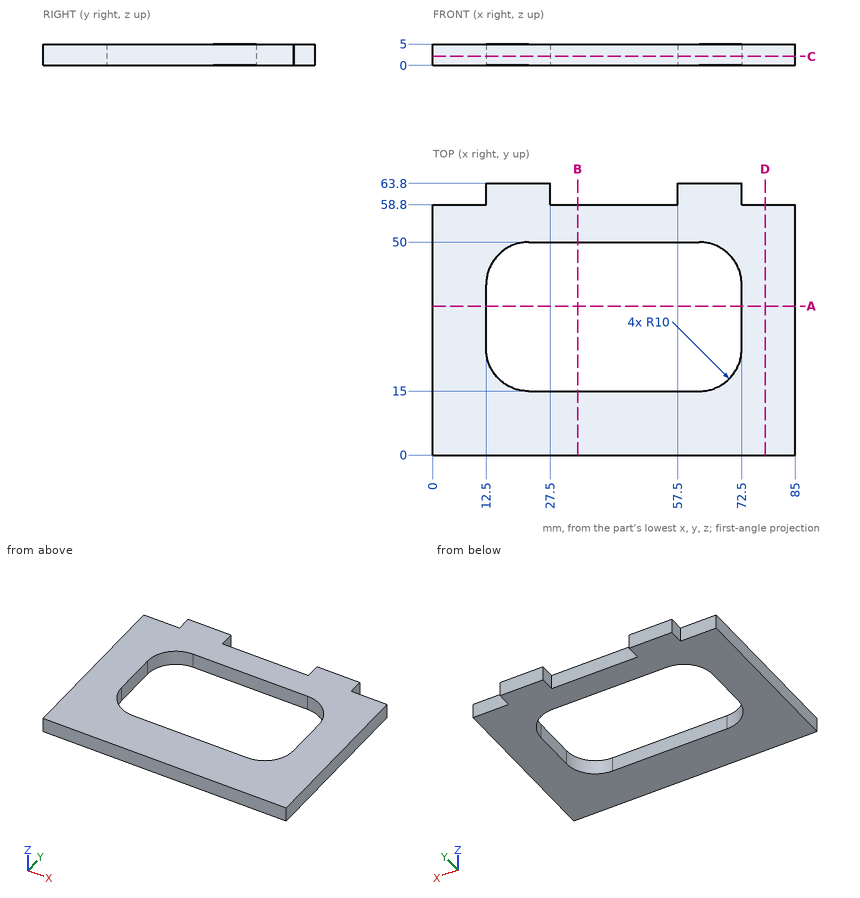
Part print with two shaded views. Sizes in mm from the minimum x, y, z corner. Coordinates: 2 decimals unless noted, no trailing zeros. Order: outer loops, then holes, each group sorted by start corner. A loop starts at its lowest first (then second) coordinate and runs counter-clockwise, first axis right, second up. Notation, with made-up numbers: (64, 33) - (119, 33) arc R16 cw to (119, 37) - close; hole circle Ø7 at (53.5, 25). An arc over 180 degrees is marked (long way). Answer in a Markdown table with one row per item.
1. Slice it at D-D, the plane x = 78. List the corners of the cut face in (y, z), then the cut area to 3 significant figures.
Answer:
| item | result |
|---|---|
| outline | (0, 0) - (58.8, 0) - (58.8, 5) - (0, 5) - close |
| area | 294 mm² |
2. Flat gauge pins, fed straight in: P1, Ø1.5, axis at x = 52.5, z = 1.5, coming from the +Y side; P2, Ø1.5, axis at y = 29, z = 2.5, coming from the -X side; P3, Ø1.5, axis at y = 61.5, z = 1.5, coming from the -X side. Where does each tip first touch, or does it go through?
Answer:
| item | result |
|---|---|
| P1 | y = 58.8 |
| P2 | x = 0 |
| P3 | x = 12.5 |
3. Drill centre lines: L1, parallel to Y at x = 35, z = 0.6; L2, parallel to Y at x = 62, z = 3.05; L3, parallel to X at y = 26, z = 3.2. Where is each one in solid material? Low to high. Write a range as from..to.
Answer:
| item | result |
|---|---|
| L1 | 0..15, 50..58.8 |
| L2 | 0..15, 50..63.8 |
| L3 | 0..12.5, 72.5..85 |
4. Slice it at A-A, the plane y = 35. List the corners of the cut face in (x, z), then the cut area to 3 significant figures.
Answer:
| item | result |
|---|---|
| outline | (0, 0) - (12.5, 0) - (12.5, 5) - (0, 5) - close; (72.5, 0) - (85, 0) - (85, 5) - (72.5, 5) - close |
| area | 125 mm² |
5. Slice it at C-C, the plane z = 2.1. List the corners of the cut face in (x, y), then the cut area to 3 significant figures.
Answer:
| item | result |
|---|---|
| outline | (0, 0) - (85, 0) - (85, 58.8) - (72.5, 58.8) - (72.5, 63.8) - (57.5, 63.8) - (57.5, 58.8) - (27.5, 58.8) - (27.5, 63.8) - (12.5, 63.8) - (12.5, 58.8) - (0, 58.8) - close; hole (12.5, 25) arc R10 ccw to (22.5, 15) - (62.5, 15) arc R10 ccw to (72.5, 25) - (72.5, 40) arc R10 ccw to (62.5, 50) - (22.5, 50) arc R10 ccw to (12.5, 40) - close |
| area | 3,130 mm² |
6. Slice it at B-B, the plane x = 34. List the corners of the cut face in (y, z), then the cut area to 3 significant figures.
Answer:
| item | result |
|---|---|
| outline | (0, 0) - (15, 0) - (15, 5) - (0, 5) - close; (50, 0) - (58.8, 0) - (58.8, 5) - (50, 5) - close |
| area | 119 mm² |
